Read the model definition and answer for the solid it produces. Units are mm, in the model's axes. Face numbers are marked on the shaded views. A direction names the side the tool comes from. Give positions to 0.01 mm unless a question says otherwise; leave off trailing zeros. Loops run counter-clockwise (first coordinate to the right, second up) from the corner with the lowest first, then second, coordinate; pieces in that order, holes last. Notation, with made-up numbers: (88, -8) - (126, -8) arc R15 ccw to (126, -2) - close; hole circle Ø2 at (-26.5, 22.25). An arc over 180 degrees is marked (long way). Write each question's results on one line, items separated by ' | '. Start each with the question number.
Q1. Given pin 1 (3 mm diameter, centred on x = 72.5, z = 45, fed in from -Y); pin 2 (8 mm diameter, centred on x = -24.5, y = 5, fed in from +Z); pin 3 (1.5 mm diameter, centred on x = 11.5, y = 43.5, fed in from +Z), each flat-ended and moving along its own axis, determine where each tip first touches the part or whether it passes through.
Q2. The part is cut by section A-A, the plane x = -12. Write down the section's boundary in (y, z), plus the area to 3 significant figures.
Q3. The part is cut by section D-D, the plane y = -37. Write down the section's boundary in (x, z).
Q4. For the marked faces 1 and 2, determine the directions among +Z, -Z, +X, -X, +Y, -Y from which every point of the face is accessible in a straight line to the end or side of a thin tool.
Q5. Find the intervals of material crossed by line 1 (X direction, y = 4, z = 3.5); line 2 (Y direction, x = 7, z = 22.5), in increasing order. Write a range as from..to.
Q6. The part is cut by section B-B, the plane z = 4.5. State how many separate pieces and enclosed holes the cut face has, plus the area to 3 significant figures.
Q7. The part is cut by section C-C, the plane z = 19.5. Write down the section's boundary in (x, y).
Q8. Determine the mould class of the marked faces 3, 4 and 5 for opening direction X: +X half, -X half, draft (parallel to the pull), parting line (faces both ways), or undercut.
Autodesk Inventor part; units mm, degrees
ref_plane "YZ Plane" through (0, 0, 0) normal (1, 0, 0) x (0, 1, 0)
ref_plane "XZ Plane" through (0, 0, 0) normal (0, 1, 0) x (-1, 0, 0)
ref_plane "XY Plane" through (0, 0, 0) normal (0, 0, 1) x (1, 0, 0)
sketch "Sketch1" plane through (0, 0, 0) normal (0, 0, 1) x (1, 0, 0)
  line L0 (-80, -80) -> (80, -80)
  line L1 (80, -80) -> (80, 80)
  line L2 (80, 80) -> (-80, 80)
  line L3 (-80, 80) -> (-80, -80)
  line L4 (-80, -80) -> (80, 80) construction
  line L5 (80, -80) -> (-80, 80) construction
  point P0 (0, 0)
  dimension "d0" = 160
  dimension "d1" = 160
extrude "Extrusion1" add sketch "Sketch1" along normal blind 60
sketch "Sketch2" plane through (0, 0, 60) normal (0, 0, 1) x (1, 0, 0)
  line L0 (-65, 65) -> (65, 65)
  line L1 (65, 65) -> (65, -65)
  line L2 (65, -65) -> (-65, -65)
  line L3 (-65, -65) -> (-65, 65)
  point P0 (0, 0)
  point P1 (-80, 80)
  point P2 (-80, -80)
  point P3 (80, -80)
extrude "Extrusion2" cut sketch "Sketch2" against normal blind 50
sketch "Sketch18" plane through (0, 0, 0) normal (0, 0, -1) x (-1, 0, 0)
  line L0 (80, 80) -> (80, -80)
  line L1 (80, 80) -> (80, -80)
  line L2 (45, 20) -> (65, 20)
  line L3 (65, 20) -> (65, -20)
  line L4 (65, -20) -> (45, -20)
  line L5 (45, -20) -> (45, 20)
  line L6 (45, 20) -> (65, -20) construction
  line L7 (65, 20) -> (45, -20) construction
  point P0 (0, 0)
  dimension "d40" = 20
  dimension "d41" = 40
extrude "Extrusion5" cut sketch "Sketch18" against normal blind 20
sketch "Sketch26" plane through (-78, 80, 0) normal (0, 1, 0) x (1, 0, 0)
  line L0 (143, -12) -> (143, -18)
  line L1 (143, -15) -> (113, -15)
  line L2 (113, -15) -> (113, -25)
  line L3 (113, -25) -> (143, -25)
  line L4 (143, -25) -> (143, -15)
  point P0 (78, 0)
  dimension "d65" = 30
  dimension "d66" = 10
extrude "Extrusion9" cut sketch "Sketch26" against normal blind 20
fillet "Fillet4" radius 2 4 edges at (65, 72.5, 25) (65, 72.5, 15) (35, 72.5, 25) (35, 72.5, 15)
sketch "Sketch36" plane through (0, 0, 10) normal (0, 0, 1) x (1, 0, 0)
  line L0 (0, -10) -> (35, -10)
  line L1 (35, -10) -> (35, 0)
  line L2 (-35, 10) -> (35, 10)
  line L3 (35, 10) -> (35, -10)
  line L4 (35, -10) -> (-35, -10)
  line L5 (-35, -10) -> (-35, 10)
  line L6 (-35, 10) -> (35, -10) construction
  line L7 (35, 10) -> (-35, -10) construction
  point P0 (0, 0)
  dimension "d75" = 10
  dimension "d76" = 35
  dimension "d77" = 10
extrude "Extrusion11" cut sketch "Sketch36" against normal blind 20
sketch "Sketch37" plane through (0, 0, 10) normal (0, 0, 1) x (1, 0, 0)
  line L0 (-49.7695, 10) -> (-40.2305, 10)
  line L1 (-40.2305, 10) -> (-40.2305, -10)
  line L2 (-40.2305, -10) -> (-49.7695, -10)
  line L3 (-49.7695, -10) -> (-49.7695, 10)
  line L4 (-45, 20) -> (-45, -20)
  line L5 (-49.7695, 10) -> (-40.2305, -10) construction
  line L6 (-40.2305, 10) -> (-49.7695, -10) construction
  point P0 (0, 0)
  point P1 (-45, 0)
  point P2 (-45, 18)
  point P3 (-45, -18)
extrude "Extrusion12" cut sketch "Sketch37" against normal blind 20
fillet "Fillet6" radius 2 4 edges at (35, 10, 5) (35, -10, 5) (-35, -10, 5) (-35, 10, 5)
fillet "Fillet7" radius 10 4 edges at (80, 80, 30) (-80, 80, 30) (-80, -80, 30) (80, -80, 30)
fillet "Fillet8" radius 2 2 edges at (-40.2305, 10, 5) (-40.2305, -10, 5)
sketch "Sketch46" plane through (0, 0, 10) normal (0, 0, 1) x (1, 0, 0)
  line L0 (-65, 20) -> (-45, 20)
  line L1 (-45, 20) -> (-45, 21)
  line L2 (-45, -20) -> (-45, -10)
  line L3 (-45, -20) -> (-45, -21)
  line L4 (-45, -21) -> (-65, -21)
  line L5 (-65, -21) -> (-65, -20)
  line L6 (-65, -20) -> (-45, -20)
  line L7 (-45, -20) -> (-45, -21)
  line L8 (-45, 21) -> (-65, 21)
  line L9 (-65, 21) -> (-65, 20)
  line L10 (-65, 20) -> (-45, 20)
  line L11 (-45, 20) -> (-45, 21)
  point P0 (0, 0)
  dimension "d87" = 1
  dimension "d88" = 1
  dimension "d89" = 20
  dimension "d90" = 1
  dimension "d91" = 20
  dimension "d92" = 1
extrude "Extrusion13" cut sketch "Sketch46" against normal blind 10
fillet "Fillet9" radius 2 4 edges at (-45, 21, 5) (-65, 21, 5) (-65, -21, 5) (-45, -21, 5)
sketch "Sketch51" plane through (80, -70, 0) normal (1, 0, 0) x (0, 0, -1)
  line L0 (-60, 5) -> (-60, 135)
  line L1 (-60, 70) -> (-45, 70)
  line L2 (-50, 52.5) -> (-40, 52.5)
  line L3 (-40, 52.5) -> (-40, 87.5)
  line L4 (-40, 87.5) -> (-50, 87.5)
  line L5 (-50, 87.5) -> (-50, 52.5)
  line L6 (-50, 52.5) -> (-40, 87.5) construction
  line L7 (-40, 52.5) -> (-50, 87.5) construction
  point P0 (0, 70)
  dimension "d103" = 15
  dimension "d104" = 10
  dimension "d105" = 35
extrude "Extrusion14" cut sketch "Sketch51" against normal blind 30
fillet "Fillet10" radius 2 4 edges at (72.5, -17.5, 40) (72.5, -17.5, 50) (72.5, 17.5, 40) (72.5, 17.5, 50)
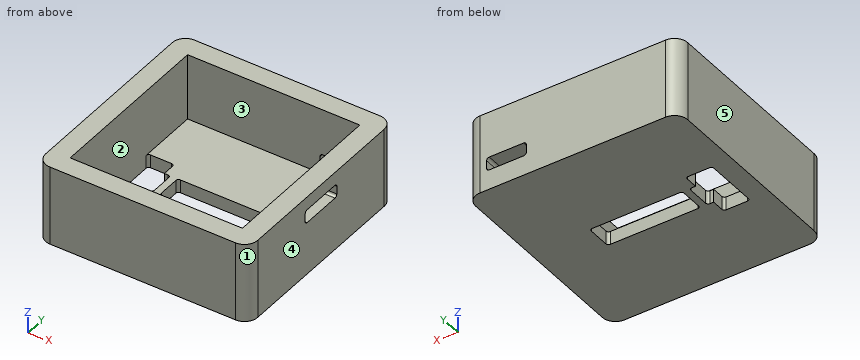
Check sheet entries:
1) pin 1: stops at y = -79.95 | pin 2: passes through | pin 3: stops at z = 10
2) outline: (-80, 0) - (-10, 0) - (-10, 10) - (-65, 10) - (-65, 60) - (-80, 60) - close; (10, 0) - (80, 0) - (80, 60) - (65, 60) - (65, 10) - (10, 10) - close | area: 2,900 mm^2
3) outline: (-80, 0) - (80, 0) - (80, 60) - (65, 60) - (65, 10) - (-65, 10) - (-65, 60) - (-80, 60) - close
4) face 1: +Z, -Z, +X, -Y | face 2: +Z
5) line 1: x = -80..-65, -40.23..-35, 35..80 | line 2: y = -80..-65, 65..80
6) separate pieces: 1 | enclosed holes: 2 | area: 23,200 mm^2
7) outline: (-80, -70) arc R10 ccw to (-70, -80) - (70, -80) arc R10 ccw to (80, -70) - (80, 70) arc R10 ccw to (70, 80) - (65, 80) - (65, -65) - (-65, -65) - (-65, 65) - (35, 65) - (35, 80) - (-70, 80) arc R10 ccw to (-80, 70) - close
8) face 3: undercut | face 4: +X half | face 5: -X half
